Here's the drawing with two shaded views (mm, measured from the low corner). I have some questions. Give positions to 0.01 mm unless a question says otherwise; leave off trailing zeros. Loops run counter-clockwise (first coordinate to the right, second up) from the corner with the lowest first, then second, coordinate; pieces in that order, holes last. Notation, with made-up numbers: (-38.75, 20) - (-20.75, 20) arc R25 ccw to (-20.75, 57) - close; hole circle Ø9 at (23, -13.5). An arc over 180 degrees is marked (long way). Answer as a JSON object with one key per item and string values. Group by question number.
Item 1: Please list where these lines run through material, in increasing order: L1, parallel to Y at x = 4.75, z = 4.3; L2, parallel to Y at x = 8.25, z = 4.1.
Item 2: Will these pins go through, and if not, where does the flat tip stop? pin 1 (0.6 mm diameter, centred on x = 4, z = 4, fed in from -Y); pin 2 (0.8 mm diameter, centred on y = 0.5, z = 4, fed in from -X) (3 decimals); pin 3 (0.5 mm diameter, centred on y = 0.5, z = 3.5, fed in from +X).
Item 3: Thinking about a two-plate mould opening in X: for the marked faces 1, 2 and 3, which applies, pulls with the +X half, pulls with the -X half, needs draft (parallel to the pull), parting line crosses it, or undercut?
Item 4: Suppose I cut it at B-B on x = 4.25. Write out the boundary of the cut face in (y, z).
Item 5: Suppose I cut it at A-A on z = 3.55. Write out the boundary of the cut face in (x, y).
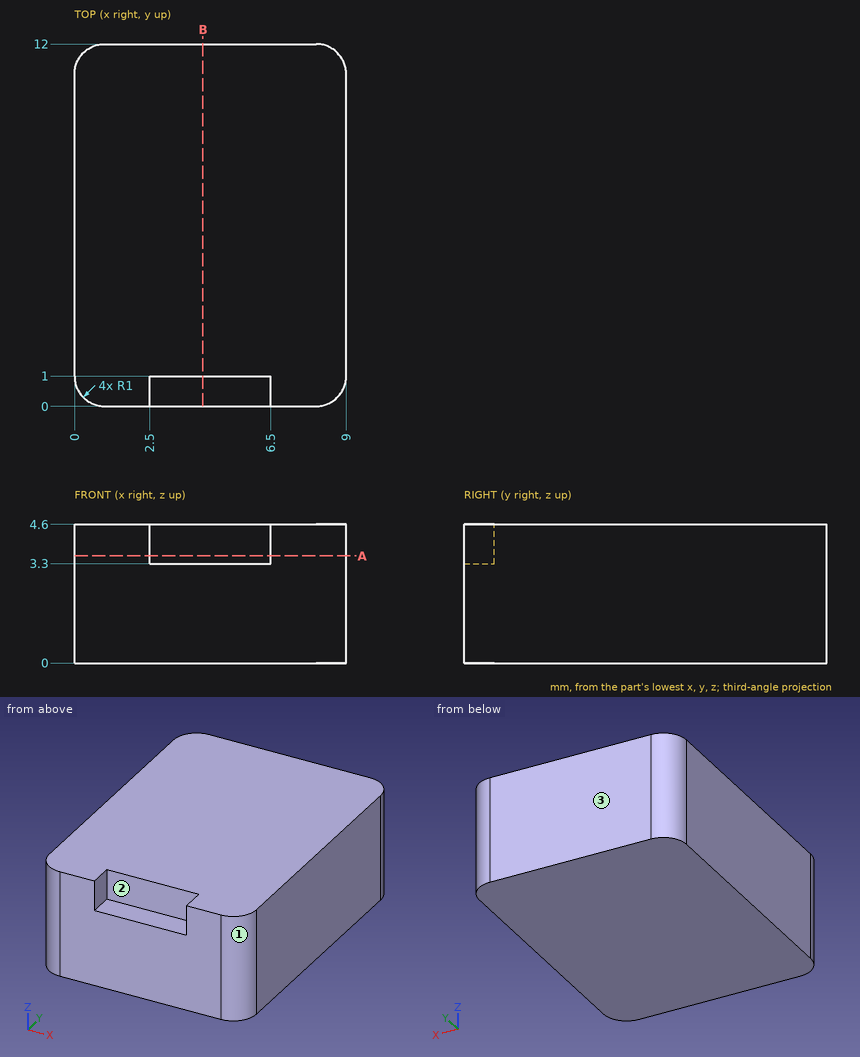
Worked out:
{
 "1": {"L1": "y = 1 to 12", "L2": "y = 0.03 to 11.97"},
 "2": {"pin 1": "stops at y = 1", "pin 2": "stops at x = 0.005", "pin 3": "stops at x = 8.97"},
 "3": {"face 1": "pulls with the +X half", "face 2": "undercut", "face 3": "needs draft"},
 "4": {"outline": "(0, 0) - (12, 0) - (12, 4.6) - (1, 4.6) - (1, 3.3) - (0, 3.3) - close"},
 "5": {"outline": "(0, 1) arc R1 ccw to (1, 0) - (2.5, 0) - (2.5, 1) - (6.5, 1) - (6.5, 0) - (8, 0) arc R1 ccw to (9, 1) - (9, 11) arc R1 ccw to (8, 12) - (1, 12) arc R1 ccw to (0, 11) - close"}
}
